For this review, use the dimensioned drawing (mm, ordinates from the lowest corner) and the shaded views. A direction names the side the tool comes from. Give positions to 0.01 mm unless a question says otherwise; leave off trailing zeros. Write each loop counter-clockwise with the first axis right and the second up, starting at its lowest first coordinate (ties: lowest second). Pieces come first, ordered by that corner, then holes.
1) We need section A-A on y = 36.5. Give the boundary of the cut face in (x, z).
2) Machinability: for the marked faces 1, 2, 3 and 4, which of the approach directions +Z, -Z, +X, -X, +Y, -Y give a long, thin tool a straight path to every point of the face, cutting with its end or side? Answer none if there is none.
3) We need section C-C on x = 11.5. Give the boundary of the cut face in (y, z).
4) For P1, Ø4, axis at y = 4, z = 4, coming from the +X side; P2, Ø8, axis at y = 20, z = 25, coming from the +X side; P3, Ø7, axis at x = 10, z = 28, coming from the -Y side; P4, Ø10.5, axis at y = 6, z = 24.5, coming from the +X side, all flat-tipped, find the tip position at first contact; note any pin that passes through.
5) We need section D-D on y = 23. Give the boundary of the cut face in (x, z).
6) We need section B-B on z = 4. Give the boundary of the cut face in (x, y).
7) Wall thickness on line 1 along Y through (x, z) = (1.55, 4); line 2 along Y through (x, z) = (9.75, 26); line 3 along Y through (x, z) = (6.25, 12): over which ranges is each line inside the solid? List them lowest first.
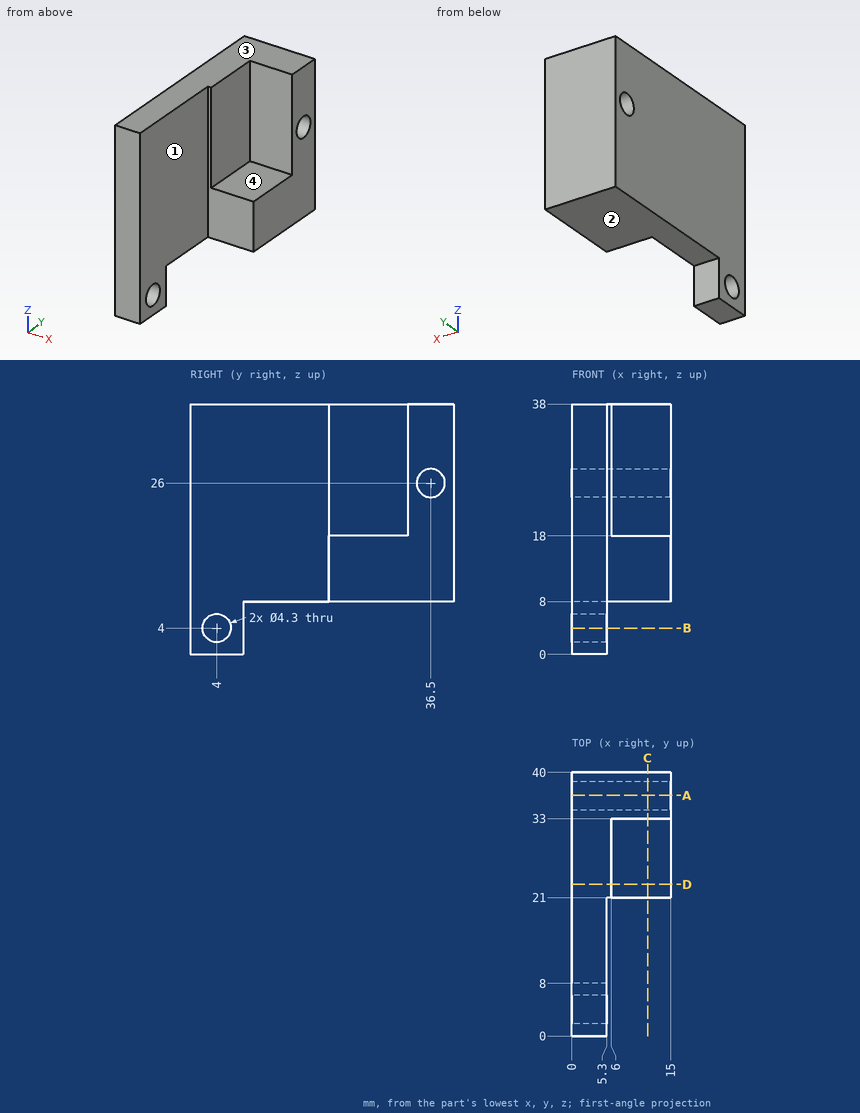
Results list:
1. outline: (0, 8) - (15, 8) - (15, 23.85) - (0, 23.85) - close; (0, 28.15) - (15, 28.15) - (15, 38) - (0, 38) - close
2. face 1: +Z, -Z, +X, -Y
2. face 2: -Z, +X, -X, +Y
2. face 3: +Z, +X, -X, +Y, -Y
2. face 4: +Z, +X, -Y
3. outline: (21, 8) - (40, 8) - (40, 38) - (33, 38) - (33, 18) - (21, 18) - close; hole circle Ø4.3 at (36.5, 26)
4. P1: passes through
4. P2: stops at x = 6
4. P3: stops at y = 33
4. P4: stops at x = 5.3
5. outline: (0, 8) - (15, 8) - (15, 18) - (6, 18) - (6, 38) - (0, 38) - close
6. outline: (0, 0) - (5.3, 0) - (5.3, 1.85) - (0, 1.85) - close; (0, 6.15) - (5.3, 6.15) - (5.3, 8) - (0, 8) - close
7. line 1: y = 0 to 1.85, 6.15 to 8
7. line 2: y = 33 to 34.35, 38.65 to 40
7. line 3: y = 21 to 40
